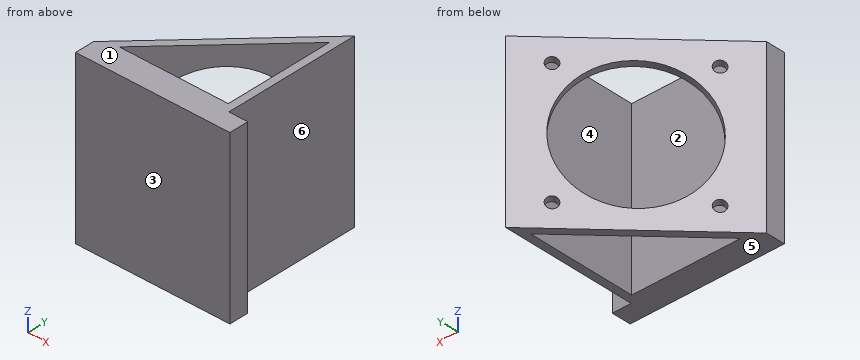
```python
from build123d import *

# Parameters (mm, degrees)
BOSS_EXTRUDE1_DEPTH = 44
CUT_EXTRUDE1_REACH  = 64.814
SKETCH2_R           = 1.5
SKETCH2_R_2         = 17
SKETCH3_W           = 40
SKETCH3_H           = 5
BOSS_EXTRUDE2_DEPTH = 44


with BuildPart() as part:
    # Sketch1 → Boss-Extrude1 (new body)
    with BuildSketch(Plane.XY):
        Polygon((2, 4.828427125), (-33.112698372, -30.284271247), (2, -30.284271247), align=None)
        Polygon((0, 0), (-28.284271247, -28.284271247), (0, -28.284271247), align=None, mode=Mode.SUBTRACT)
    extrude(amount=BOSS_EXTRUDE1_DEPTH)

    # Sketch2 → Cut-Extrude1 (cut, up to next)
    with BuildSketch(Plane(origin=(-1.414213562, 1.414213562, 0), x_dir=(0, 0, 1), z_dir=(-0.7071067811865513, 0.7071067811865437, 0)), mode=Mode.PRIVATE) as cut_extrude1_sk1:
        with Locations(Location((6, -36, 0), (0, 0, 270))):
            Circle(SKETCH2_R)
    cut_extrude1_tool1 = extrude(cut_extrude1_sk1.sketch, amount=-CUT_EXTRUDE1_REACH, mode=Mode.PRIVATE) & part.part
    # Sketch2 → Cut-Extrude1 (cut, up to next)
    with BuildSketch(Plane(origin=(-1.414213562, 1.414213562, 0), x_dir=(0, 0, 1), z_dir=(-0.7071067811865513, 0.7071067811865437, 0)), mode=Mode.PRIVATE) as cut_extrude1_sk2:
        with Locations(Location((6, -4, 0), (0, 0, 270))):
            Circle(SKETCH2_R)
    cut_extrude1_tool2 = extrude(cut_extrude1_sk2.sketch, amount=-CUT_EXTRUDE1_REACH, mode=Mode.PRIVATE) & part.part
    # Sketch2 → Cut-Extrude1 (cut, up to next)
    with BuildSketch(Plane(origin=(-1.414213562, 1.414213562, 0), x_dir=(0, 0, 1), z_dir=(-0.7071067811865513, 0.7071067811865437, 0)), mode=Mode.PRIVATE) as cut_extrude1_sk3:
        with Locations(Location((38, -36, 0), (0, 0, 270))):
            Circle(SKETCH2_R)
    cut_extrude1_tool3 = extrude(cut_extrude1_sk3.sketch, amount=-CUT_EXTRUDE1_REACH, mode=Mode.PRIVATE) & part.part
    # Sketch2 → Cut-Extrude1 (cut, up to next)
    with BuildSketch(Plane(origin=(-1.414213562, 1.414213562, 0), x_dir=(0, 0, 1), z_dir=(-0.7071067811865513, 0.7071067811865437, 0)), mode=Mode.PRIVATE) as cut_extrude1_sk4:
        with Locations(Location((38, -4, 0), (0, 0, 270))):
            Circle(SKETCH2_R)
    cut_extrude1_tool4 = extrude(cut_extrude1_sk4.sketch, amount=-CUT_EXTRUDE1_REACH, mode=Mode.PRIVATE) & part.part
    # Sketch2 → Cut-Extrude1 (cut, up to next)
    with BuildSketch(Plane(origin=(-1.414213562, 1.414213562, 0), x_dir=(0, 0, 1), z_dir=(-0.7071067811865513, 0.7071067811865437, 0)), mode=Mode.PRIVATE) as cut_extrude1_sk5:
        with Locations(Location((22, -20, 0), (0, 0, 270))):
            Circle(SKETCH2_R_2)
    cut_extrude1_tool5 = extrude(cut_extrude1_sk5.sketch, amount=-CUT_EXTRUDE1_REACH, mode=Mode.PRIVATE) & part.part
    add(cut_extrude1_tool1.solids().sort_by_distance((-26.870058, -24.041631, 6))[0], mode=Mode.SUBTRACT)
    add(cut_extrude1_tool2.solids().sort_by_distance((-4.242641, -1.414214, 6))[0], mode=Mode.SUBTRACT)
    add(cut_extrude1_tool3.solids().sort_by_distance((-26.870058, -24.041631, 38))[0], mode=Mode.SUBTRACT)
    add(cut_extrude1_tool4.solids().sort_by_distance((-4.242641, -1.414214, 38))[0], mode=Mode.SUBTRACT)
    add(cut_extrude1_tool5.solids().sort_by_distance((-15.556349, -12.727922, 22))[0], mode=Mode.SUBTRACT)

    # Sketch3 → Boss-Extrude2 (add)
    with BuildSketch(Plane.XY):
        with Locations((-13.112698372, -32.784271247)):
            Rectangle(SKETCH3_W, SKETCH3_H)
    extrude(amount=BOSS_EXTRUDE2_DEPTH)


solid = part.part
```
Design review of the part built by this model. Coordinates are the model's own, in mm. Face numbers are marked on the shaded views. A direction names the side the tool comes from. Round coordinates to 2 decimals unless told otherwise and drop trailing zeros. Write each loop counter-clockwise with the first axis right and the second up, starting at its lowest first coordinate (ties: lowest second). Pieces come first, ordered by that corner, then holes. Notation, with made-up numbers: (41.5, -20) -> (94.5, -20) arc R11 ccw to (94.5, -8) -> close; hole circle Ø1 at (-23, 39.5). An arc over 180 degrees is marked (long way). Write item = value, one per line. Start each with the question number.
1) Take a section at A-A, the plane z = 16. State the section outline as (x, y) points.
2) Tool access review of the marked faces 4, 5 and 6: name each direction out of +Z, -Z, +X, -X, +Y, -Y from which nothing blocks a thin tool from reaching the whole face with its end or side.
3) Mouldability with a two-part tool opening along Y and no side actions: class the marked faces 1, 2 and 3 as +Y half, -Y half, draft (parallel to the pull), parting line (faces both ways), or undercut.
4) Clearance check with flat-ended pins moving along their axes: pin 1 (8 mm diameter, centred on x = -13, y = -9.5, fed in from +Z); pin 2 (5.5 mm diameter, centred on x = 5, z = 25.5, fed in from +Y); pin 3 (22.5 mm diameter, centred on y = -13.5, z = 20.5, fed in from -X); pin 4 (10 mm diameter, centred on y = -24, z = 17, fed in from -X). State where each tip first meets the part, or that it passes through.
5) Wall thickness on probe 1 along X at (y, z) = (-12.5, 29.5); probe 2 along Y at (x, z) = (-24.5, 40.5); probe 3 along Y at (x, z) = (-4.5, 37): over which ranges is each line inside the solid? List them lowest first. Write a range as from..to.
6) Take a section at B-B, the plane y = -16.5. Count the separate pieces of the cut face and the enclosed holes in it, plus the area to 3 significant figures.
7) Take a section at D-D, the plane z = 31. State the section outline as (x, y) points.
Results list:
q1.outline = (-33.11, -35.28) -> (6.89, -35.28) -> (6.89, -30.28) -> (2, -30.28) -> (2, 4.83) -> (-4.31, -1.48) -> (-2.89, -2.89) -> (0, 0) -> (0, -28.28) -> (-28.28, -28.28) -> (-25.39, -25.39) -> (-26.8, -23.98) -> (-33.11, -30.28) -> close
q2.face_4 = +Z, -Z
q2.face_5 = -Z, +X, -X, +Y, -Y
q2.face_6 = +Z, -Z, +X, +Y
q3.face_1 = draft
q3.face_2 = undercut
q3.face_3 = -Y half
q4.pin_1 = 44
q4.pin_2 = -30.28
q4.pin_3 = -27.58
q4.pin_4 = -31.83
q5.probe_1 = 0..2
q5.probe_2 = -35.28..-28.28, -24.5..-21.67
q5.probe_3 = -35.28..-28.28, -4.5..-2.74
q6.separate_pieces = 3
q6.enclosed_holes = 0
q6.area = 120 mm²
q7.outline = (-33.11, -35.28) -> (6.89, -35.28) -> (6.89, -30.28) -> (2, -30.28) -> (2, 4.83) -> (-5.36, -2.53) -> (-3.94, -3.94) -> (0, 0) -> (0, -28.28) -> (-28.28, -28.28) -> (-24.34, -24.34) -> (-25.75, -22.93) -> (-33.11, -30.28) -> close
